Autodesk Inventor part; units mm, degrees
ref_plane "YZ Plane" through (0, 0, 0) normal (1, 0, 0) x (0, 1, 0)
ref_plane "XZ Plane" through (0, 0, 0) normal (0, 1, 0) x (-1, 0, 0)
ref_plane "XY Plane" through (0, 0, 0) normal (0, 0, 1) x (1, 0, 0)
sketch "Эскиз1" plane through (0, 0, 0) normal (1, 0, 0) x (0, 1, 0)
  circle A0 centre (35.2311, -22.6062) radius 9.3
  circle A1 centre (0, -38.8201) radius 6.1
  circle A2 centre (0, 0) radius 4.85
  circle A3 centre (35.8147, -49.5529) radius 3.55
  line L0 (6.0968, -38.6237) -> (4.8475, 0.1562)
  line L1 (-4.8475, 0.1562) -> (-6.0968, -38.6237)
  line L2 (0, 0) -> (0, -38.8201) construction
  circle A4 centre (0, -38.8201) radius 6.5
  circle A5 centre (0, 0) radius 2
  circle A6 centre (0, -38.8201) radius 15 construction
  circle A7 centre (0, 0) radius 14 construction
  circle A8 centre (0, -38.8201) radius 9.5
  circle A9 centre (0, 0) radius 7
  line L3 (9.4833, -39.383) -> (11.7793, -0.6991)
  line L4 (-9.4833, -39.383) -> (-11.7793, -0.6991)
  circle A10 centre (0, 0) radius 8.8
  circle A11 centre (0, 0) radius 11.8
  point P0 (-7, 0)
  point P1 (-9.4833, -39.383)
  point P2 (-11.7793, -0.6991)
  dimension "d27" = 19
  dimension "d0" = 18.6
  dimension "d1" = 12.2
  dimension "d2" = 9.7
  dimension "d3" = 7.1
  dimension "d8" = 38.8201
  dimension "d13" = 38.8
  dimension "d14" = 38.8
  dimension "d23" = 13
  dimension "d24" = 4
  dimension "d25" = 30
  dimension "d26" = 28
  dimension "d28" = 14
  dimension "d31" = 17.6
  dimension "d32" = 3
extrude "Выдавливание4" add sketch "Эскиз1" along normal blind 3 contours A4 L1 A8 L0 | L0 A8 L1 A4 | A8 L1 A11 L0 | L0 A11 L3 A8 | A8 L4 A11 L1 | A11 L1 A10 L0 | L0 A10 L1 A11 | A10 L1 A9 L0 | L0 A9 L1 A10 | A9 L1 A2 L0 | L0 A2 L1 A9 | A2
sketch "Эскиз4" plane through (0, 0, 0) normal (-1, 0, 0) x (0, 0, 1)
  circle A0 centre (-6.2, 6.2) radius 1.25
  circle A1 centre (0, 0) radius 2 construction
  circle A2 centre (-38.8201, 0) radius 6.5 construction
  arc A3 (-0.6991, -11.7793) -> (-0.6991, 11.7793) centre (0, 0) ccw construction
  line L0 (-39.383, 9.4833) -> (-0.6991, 11.7793) construction
  arc A4 (-39.383, 9.4833) -> (-39.383, -9.4833) centre (-38.8201, 0) ccw construction
  line L1 (-0.6991, -11.7793) -> (-39.383, -9.4833) construction
  line L2 (0, 0) -> (0, 11.8) construction
  arc A5 (-0.6991, -11.7793) -> (-0.6991, 11.7793) centre (0, 0) ccw construction
  line L3 (0, 0) -> (11.8, 0) construction
  circle A6 centre (6.2, 6.2) radius 1.25
  circle A7 centre (-6.2, -6.2) radius 1.25
  circle A8 centre (6.2, -6.2) radius 1.25
  dimension "d33" = 2.5
  dimension "d34" = 12.4
  dimension "d35" = 12.4
extrude "Выдавливание5" cut sketch "Эскиз4" against normal blind 3
sketch "Эскиз5" plane through (3, 0, 0) normal (1, 0, 0) x (0, 0, -1)
  circle A0 centre (0, 0) radius 3.5
  dimension "d38" = 7
extrude "Выдавливание6" cut sketch "Эскиз5" against normal blind 1
sketch "Эскиз6" plane through (3, 0, 0) normal (1, 0, 0) x (0, 0, -1)
  circle A0 centre (0, -18) radius 2
  circle A1 centre (0, 0) radius 3.5 construction
  circle A2 centre (-6.2, -6.2) radius 1.25 construction
  circle A3 centre (-6.2, 6.2) radius 1.25 construction
  circle A4 centre (6.2, -6.2) radius 1.25 construction
  circle A5 centre (6.2, 6.2) radius 1.25 construction
  circle A6 centre (38.8201, 0) radius 6.5 construction
  line L0 (39.383, 9.4833) -> (0.6991, 11.7793) construction
  arc A7 (0.6991, 11.7793) -> (0.6991, -11.7793) centre (0, 0) ccw construction
  line L1 (0.6991, -11.7793) -> (39.383, -9.4833) construction
  arc A8 (39.383, -9.4833) -> (39.383, 9.4833) centre (38.8201, 0) ccw construction
  line L2 (0, 0) -> (0, -26.6004) construction
  circle A9 centre (0, 0) radius 14 construction
  line L3 (-10.6346, -5.1133) -> (-3.6049, -19.7333)
  arc A10 (0, -14) -> (-3.6049, -19.7333) centre (0, -18) ccw construction
  line L4 (2.8284, -20.8284) -> (12.5829, -11.0739)
  line L5 (0.6991, -11.7793) -> (39.383, -9.4833) construction
  arc A11 (2.8284, -20.8284) -> (0, -14) centre (0, -18) ccw construction
  arc A12 (-3.6049, -19.7333) -> (2.8284, -20.8284) centre (0, -18) ccw
  line L6 (-10.6346, -5.1133) -> (-9.9206, -5.1133)
  line L7 (-9.9206, -5.1133) -> (-6.5876, -8.9793)
  line L8 (-6.5876, -8.9793) -> (5.3497, -10.0676)
  line L9 (5.3497, -10.0676) -> (12.5829, -11.0739)
  dimension "d42" = 28
  dimension "d41" = 4
  dimension "d43" = 18
  dimension "d44" = 8
  dimension "d45" = 45
extrude "Выдавливание7" [suppressed]
sketch "Эскиз7" plane through (3, 0, 0) normal (1, 0, 0) x (0, 0, -1)
  line L0 (0, 0) -> (0, -29.4139) construction
  circle A0 centre (-7.6071, -16.3135) radius 2
  line L1 (-7.6071, -16.3135) -> (0, 0) construction
  circle A1 centre (0, 0) radius 14 construction
  circle A2 centre (0, 0) radius 18 construction
  arc A3 (-6.239, -20.0723) -> (-11.6068, -16.361) centre (-7.6071, -16.3135) ccw construction
  circle A4 centre (0, 0) radius 3.5 construction
  circle A5 centre (-6.2, -6.2) radius 1.25 construction
  circle A6 centre (-6.2, 6.2) radius 1.25 construction
  circle A7 centre (6.2, -6.2) radius 1.25 construction
  circle A8 centre (6.2, 6.2) radius 1.25 construction
  circle A9 centre (38.8201, 0) radius 6.5 construction
  line L2 (39.383, 9.4833) -> (0.6991, 11.7793) construction
  arc A10 (0.6991, 11.7793) -> (0.6991, -11.7793) centre (0, 0) ccw
  line L3 (0.6991, -11.7793) -> (39.383, -9.4833)
  arc A11 (39.383, -9.4833) -> (39.383, 9.4833) centre (38.8201, 0) ccw construction
  line L4 (-11.7992, -0.1399) -> (-11.6068, -16.361)
  line L5 (-6.239, -20.0723) -> (19.6335, -10.6555)
  line L6 (0.6991, -11.7793) -> (39.383, -9.4833) construction
  arc A12 (-11.6068, -16.361) -> (-6.239, -20.0723) centre (-7.6071, -16.3135) ccw
  point P0 (19.6335, -10.6555)
  dimension "d48" = 4
  dimension "d50" = 28
  dimension "d52" = 8
  dimension "d53" = 45
  dimension "d56" = 25
  dimension "d57" = 4
extrude "Выдавливание8" add sketch "Эскиз7" against normal up to surface (3 mm away)
properties part number "right_wall"
Work out the finished part from the listing and answer in its coordinate system (mm). A direction names the side the tool comes from. Give positions to 0.01 mm unless a question says otherwise; leave off trailing zeros. Order: outer loops, then holes, each group sorted by start corner. A loop starts at its lowest first (then second) coordinate and runs counter-clockwise, first axis right, second up. Notation, with made-up numbers: (-33, 58.5) - (11, 58.5) arc R30 cw to (11, 92.5) - close; hole circle Ø11 at (71.5, 56). An arc over 180 degrees is marked (long way). Answer as CSV lines item,"result". Start each with the question number.
Q1. The part is cut by section A-A (z = -33). Write down the section's boundary in (x, y), then the cut area to 3 significant figures.
Q2. The part is cut by section C-C (x = 0.6). Write down the section's boundary in (y, z), then the cut area to 3 significant figures.
Q3. For faces 1 (the face through (1.48, -6.15, -7.45)), 2 (the face through (2.507, -1.341, -3.233)), determine the directions among +Z, -Z, +X, -X, +Y, -Y from which every point of the face is accessible in a straight line to the end or side of a thin tool.
Q4. Find the intervals of material crossed by L1, parallel to Z at x = 1.1, y = 0; L2, parallel to Z at x = 1.45, y = 6; L3, parallel to Y at x = 2.25, z = -37, in increasing order. Write a range as [from, to].
Q5. The mould has two halves that part along Y. Classify faces 3 (the face through (3, 0, -11)), 4 (the face through (1.48, -10.06, -29.65)), 5 (the face through (1.48, 7.44, -6.36)): +Y half, -Y half, draft (parallel to the pull), parting line (faces both ways), or undercut.
Q6. The part is cut by section B-B (y = -17.5). Write down the section's boundary in (x, z).
Q7. The part is cut by section D-D (z = -6.2). Write down the section's boundary in (x, y), then the cut area to 3 significant figures.
Check result:
1,outline,"(0, -9.86) - (3, -9.86) - (3, -2.89) - (0, -2.89) - close; (0, 2.89) - (3, 2.89) - (3, 9.86) - (0, 9.86) - close"
1,area,"41.8 mm²"
2,outline,"(-20.07, 6.24) - (-10.66, -19.63) - (-9.48, -39.38) arc R9.5 ccw to (9.48, -39.38) - (11.78, -0.7) arc R11.8 ccw to (-0.14, 11.8) - (-16.36, 11.61) arc R4 ccw to start; hole circle Ø4 at (-16.31, 7.61); hole circle Ø2.5 at (-6.2, -6.2); hole circle Ø2.5 at (-6.2, 6.2); hole circle Ø13 at (0, -38.82); hole circle Ø4 at (0, 0); hole circle Ø2.5 at (6.2, -6.2); hole circle Ø2.5 at (6.2, 6.2)"
2,area,"1,190 mm²"
3,face 1,"+X, -X"
3,face 2,"+X"
4,L1,"z = [-48.32, -45.32], [-32.32, -2], [2, 11.8]"
4,L2,"z = [-46.19, -41.32], [-36.32, -7.43], [-4.97, 4.97], [7.43, 10.16]"
4,L3,"y = [-9.62, -6.24], [6.24, 9.62]"
5,face 3,"draft"
5,face 4,"-Y half"
5,face 5,"undercut"
6,outline,"(0, -0.83) - (3, -0.83) - (3, 6) - (0, 6) - close; (0, 9.22) - (3, 9.22) - (3, 11.43) - (0, 11.43) - close"
7,outline,"(0, -15.54) - (3, -15.54) - (3, -7.45) - (0, -7.45) - close; (0, -4.95) - (3, -4.95) - (3, 4.95) - (0, 4.95) - close; (0, 7.45) - (3, 7.45) - (3, 11.45) - (0, 11.45) - close"
7,area,"66.0 mm²"
